Source: three-view drawing plus pictorial views. Frame: mm from the lowest corner of the part. A direction names the side the tool comes from. Round coordinates to 2 decimals unless told otherwise and drop trailing zeros. Loops run counter-clockwise (first coordinate to the right, second up) from the corner with the lowest first, then second, coordinate; pieces in that order, holes last. Notation, with made-up numbers: (8.5, 12.25) -> (40.5, 12.25) arc R33 cw to (40.5, 50.25) -> close; hole circle Ø4 at (38, 3.5). An arc over 180 degrees is marked (long way). Answer as a JSON object with one key per item and string values. Group by question number.
Item 1: Draft query along X for the marked faces 1, 2 and 3. Return one class per face: released by +X, released by -X, zero draft, split by the parting line, or undercut.
Item 2: Pin query (flat end, axial travel): pin 1 (3.5 mm diameter, centred on y = 9.25, z = 96.04, fed in from +X); pin 2 (6 mm diameter, centred on x = 34.57, z = 44.17, fed in from +Y). Return the tip coordinate at first contact, or that it passes through.
Item 3: Material intervals for line 1 (X direction, y = 14, z = 68); line 2 (Y direction, x = 39, z = 84); line 3 (X direction, y = 3.25, z = 60) (1 decimal), sorted ascending. Write a range as [from, to].
Item 4: Set-up query: the marked faces 4 and 5. Return all of +Z, -Z, +X, -X, +Y, -Y with unobstructed straight access to the full face (end or side cutting, diameter ignored); none if empty.
Item 5: Section query B-B on y = 12.25. Return loops of the section in (x, z).
Item 6: Section query C-C on x = 44. Return loops of the section in (y, z).
Item 7: Section query A-A on z = 53. Return loops of the section in (x, y) (1 decimal).
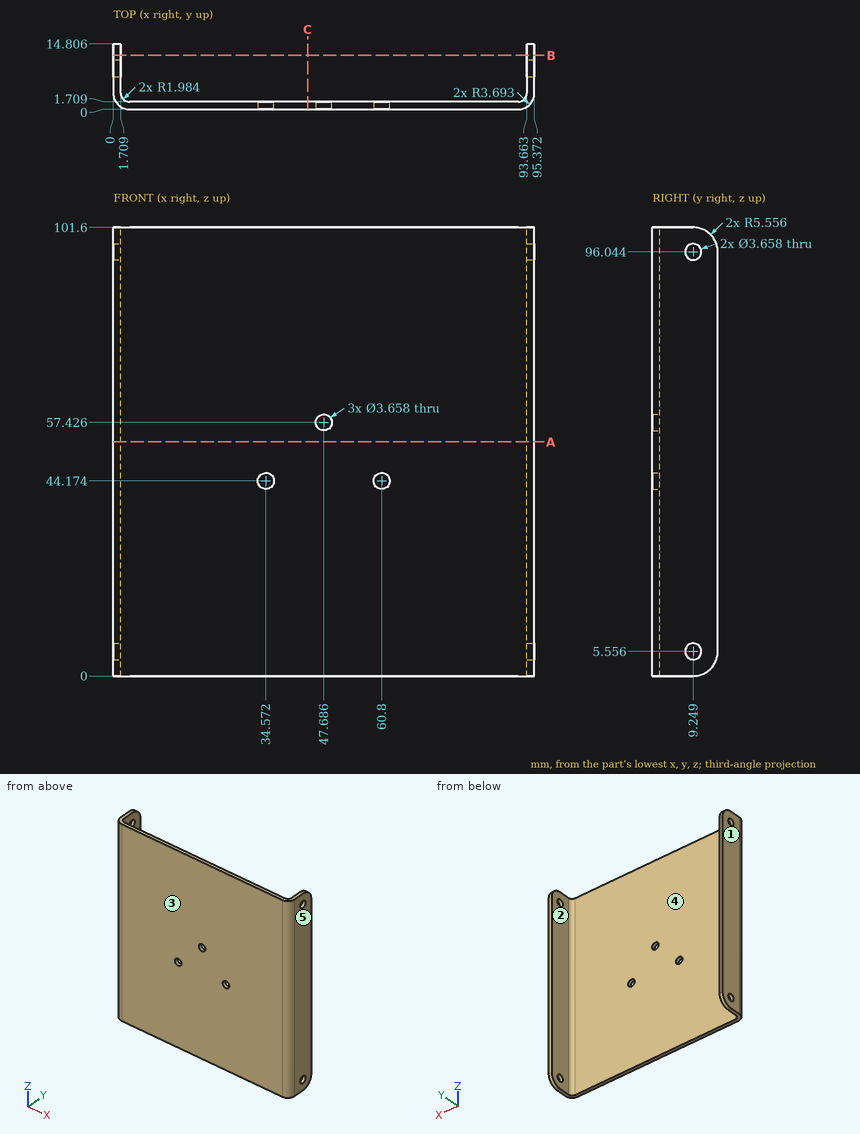
Solved:
{
 "1": {"face 1": "released by -X", "face 2": "undercut", "face 3": "zero draft"},
 "2": {"pin 1": "through", "pin 2": "y = 1.71"},
 "3": {"line 1": "[0, 1.71], [93.66, 95.37]", "line 2": "[0, 1.71]", "line 3": "[0, 1.8], [93.6, 95.3]"},
 "4": {"face 4": "+Z, -Z, +Y", "face 5": "+Z, -Z, +X, +Y, -Y"},
 "5": {"outline": "(0, 0.88) -> (1.71, 0.88) -> (1.71, 100.72) -> (0, 100.72) -> close; (93.66, 0.88) -> (95.37, 0.88) -> (95.37, 100.72) -> (93.66, 100.72) -> close"},
 "6": {"outline": "(0, 0) -> (1.71, 0) -> (1.71, 101.6) -> (0, 101.6) -> close"},
 "7": {"outline": "(0, 3.7) arc R3.7 ccw to (3.7, 0) -> (91.7, 0) arc R3.7 ccw to (95.4, 3.7) -> (95.4, 14.8) -> (93.7, 14.8) -> (93.7, 3.7) arc R2 cw to (91.7, 1.7) -> (3.7, 1.7) arc R2 cw to (1.7, 3.7) -> (1.7, 14.8) -> (0, 14.8) -> close"}
}
